Work out the finished part from the listing and answer in its coordinate system (mm). Face numbers are marked on the shaded views. A direction names the side the tool comes from. Round coordinates to 2 decimals unless told otherwise and drop trailing zeros. Order: outer loops, then holes, each group sorted by start corner. A loop starts at its lowest first (then second) coordinate and runs counter-clockwise, first axis right, second up. Notation, with made-up numbers: (-25, 62) -> (-5, 62) arc R6 ccw to (-5, 70) -> close; hole circle Ø9 at (66.5, 41.25). An arc over 180 degrees is marked (long way). Use one line per item in the form item = value.
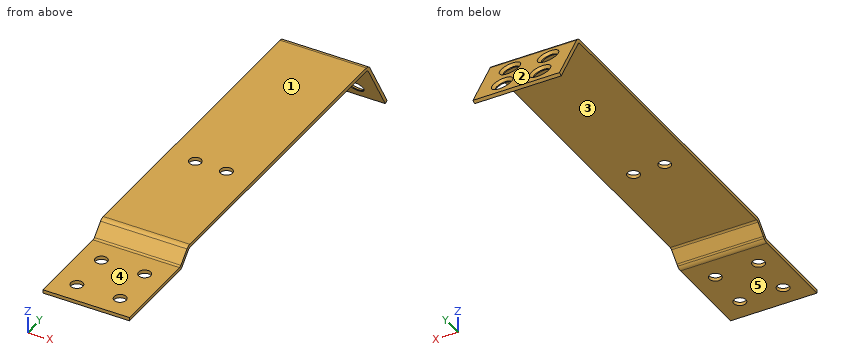
```python
from build123d import *

# Parameters (mm, degrees)
SKETCH_1_W                            = 50
SKETCH_1_H                            = 245
SM_BASE_FLANGE_1_DEPTH                = 2
SM_START                              = -25
SM_EDGE_FLANGE_1_DEPTH                = 50
SM_EDGE_FLANGE_1_2_DEPTH              = 50
OTHER_START                           = -25
OTHER_1_DEPTH                         = 50
OTHER_1_2_DEPTH                       = 50
HOLE_WIZARD_M61_D                     = 9
HOLE_WIZARD_M61_CSINK_D               = 12
HOLE_WIZARD_M61_CSINK_ANGLE           = 90
HOLE_WIZARD_M61_ON_FACE_2_D           = 9
HOLE_WIZARD_M61_ON_FACE_2_CSINK_D     = 12
HOLE_WIZARD_M61_ON_FACE_2_CSINK_ANGLE = 90
HOLE_WIZARD_M61_ON_FACE_3_D           = 9
HOLE_WIZARD_M61_ON_FACE_3_CSINK_D     = 12
HOLE_WIZARD_M61_ON_FACE_3_CSINK_ANGLE = 90
SKETCH_9_R                            = 3.5
CUT_EXTRUDE_1_DEPTH                   = 2
SKETCH_10_R                           = 3.5
CUT_EXTRUDE_2_DEPTH                   = 2


# Read off the part's stored shape, not the designer's step: Ребро-кромка1, Изгиб1
# Sheet-metal steps are written as plain solids
with BuildPart() as part:
    # Sketch 1 → Базовая кромка1 (new body)
    with BuildSketch(Plane.XY):
        with Locations((0, 122.5)):
            Rectangle(SKETCH_1_W, SKETCH_1_H)
    extrude(amount=SM_BASE_FLANGE_1_DEPTH)

    # Ребро-кромка1 outline → Ребро-кромка1 (cut)
    with BuildSketch(Plane.YZ.offset(SM_START)):
        with BuildLine():
            ThreePointArc((241.535898385, 2), (243.535898385, 1.464101615), (245, 0))
            Line((245, 0), (245, 2))
            Line((245, 2), (241.535898385, 2))
        make_face()
    extrude(amount=SM_EDGE_FLANGE_1_DEPTH, mode=Mode.SUBTRACT)

    # Sm Edge Flange 1 2 outline → Sm Edge Flange 1 2 (add)
    with BuildSketch(Plane.YZ.offset(SM_START)):
        with BuildLine():
            Line((262.422649731, -30.176914536), (245, 0))
            Line((245, 0), (241.535898385, 0))
            ThreePointArc((241.535898385, 0), (242.535898385, -0.267949192), (243.267949192, -1))
            Line((243.267949192, -1), (260.690598923, -31.176914536))
            Line((260.690598923, -31.176914536), (262.422649731, -30.176914536))
        make_face()
    extrude(amount=SM_EDGE_FLANGE_1_2_DEPTH)

    # Other 1 outline → Other 1 (cut)
    with BuildSketch(Plane.YZ.offset(OTHER_START)):
        with BuildLine():
            Line((241.535898385, 2), (54.65685425, 2))
            Line((54.65685425, 2), (53.82842715, 1.17157285))
            ThreePointArc((53.82842715, 1.17157285), (52.530733743, 0.304481837), (51, -3.6e-08))
            Line((51, -3.6e-08), (241.535898385, 0))
            ThreePointArc((241.535898385, 0), (242.535898385, -0.267949192), (243.267949192, -1))
            Line((243.267949192, -1), (260.690598923, -31.176914536))
            Line((260.690598923, -31.176914536), (262.422649731, -30.176914536))
            Line((262.422649731, -30.176914536), (245, 0))
            ThreePointArc((245, 0), (243.535898385, 1.464101615), (241.535898385, 2))
        make_face()
    extrude(amount=OTHER_1_DEPTH, mode=Mode.SUBTRACT)

    # Other 1 2 outline → Other 1 2 (add)
    with BuildSketch(Plane.YZ.offset(OTHER_START)):
        with BuildLine():
            Line((241.535898385, 10), (61.485281398, 10.000000033))
            ThreePointArc((61.485281398, 10.000000033), (59.954547643, 9.695518165), (58.656854226, 8.828427148))
            Line((58.656854226, 8.828427148), (52.414213588, 2.585786412))
            ThreePointArc((52.414213588, 2.585786412), (51.765366878, 2.152240902), (51, 1.999999964))
            Line((51, 1.999999964), (54.65685425, 2))
            Line((54.65685425, 2), (60.071067788, 7.414213586))
            ThreePointArc((60.071067788, 7.414213586), (60.719914496, 7.847759096), (61.485281374, 8.000000033))
            Line((61.485281374, 8.000000033), (241.535898385, 8))
            ThreePointArc((241.535898385, 8), (242.535898385, 7.732050808), (243.267949192, 7))
            Line((243.267949192, 7), (260.690598923, -23.176914536))
            Line((260.690598923, -23.176914536), (262.422649731, -22.176914536))
            Line((262.422649731, -22.176914536), (245, 8))
            ThreePointArc((245, 8), (243.535898385, 9.464101615), (241.535898385, 10))
        make_face()
    extrude(amount=OTHER_1_2_DEPTH)

    # Зенковка для винта с потайной головкой M61 (through all)
    with Locations(Plane(origin=(-11, 257.422649731, -13.516660498), x_dir=(0, -0.5, 0.866025403784), z_dir=(0, 0.866025403784, 0.5))):
        with Locations((0, 0)):
            CounterSinkHole(HOLE_WIZARD_M61_D / 2, HOLE_WIZARD_M61_CSINK_D / 2, counter_sink_angle=HOLE_WIZARD_M61_CSINK_ANGLE)

    # Зенковка для винта с потайной головкой M61 on face 2 (through all)
    with Locations(Plane(origin=(11, 257.422649731, -13.516660498), x_dir=(0, -0.500000174844, 0.866025302838), z_dir=(0, 0.866025302838, 0.500000174844))):
        with Locations((0, 0)):
            CounterSinkHole(HOLE_WIZARD_M61_ON_FACE_2_D / 2, HOLE_WIZARD_M61_ON_FACE_2_CSINK_D / 2, counter_sink_angle=HOLE_WIZARD_M61_ON_FACE_2_CSINK_ANGLE)

    # Зенковка для винта с потайной головкой M61 on face 3 (through all)
    with Locations(Plane(origin=(11, 249.422649731, 0.339745962), x_dir=(0, -0.500000174844, 0.866025302838), z_dir=(0, 0.866025302838, 0.500000174844))):
        with Locations((0, 0), (0, -22)):
            CounterSinkHole(HOLE_WIZARD_M61_ON_FACE_3_D / 2, HOLE_WIZARD_M61_ON_FACE_3_CSINK_D / 2, counter_sink_angle=HOLE_WIZARD_M61_ON_FACE_3_CSINK_ANGLE)

    # Эскиз9 → Вытянуть1 (cut)
    with BuildSketch(Plane.XY.offset(2)):
        with Locations((-12.5, 37.5)):
            Circle(SKETCH_9_R)
        with Locations((-12.5, 12.5)):
            Circle(SKETCH_9_R)
        with Locations((12.5, 12.5)):
            Circle(SKETCH_9_R)
        with Locations((12.5, 37.5)):
            Circle(SKETCH_9_R)
    extrude(amount=-CUT_EXTRUDE_1_DEPTH, mode=Mode.SUBTRACT)

    # Эскиз10 → Вытянуть2 (cut)
    with BuildSketch(Plane.XY.offset(10)):
        with Locations((-9, 127)):
            Circle(SKETCH_10_R)
        with Locations((9, 127)):
            Circle(SKETCH_10_R)
    extrude(amount=-CUT_EXTRUDE_2_DEPTH, mode=Mode.SUBTRACT)


solid = part.part
```
Item 1: Consider line 1 along X through (y, z) = (12, 1); line 2 along Y through (x, z) = (-12, 1); line 3 along Y through (x, z) = (12.5, 0.65). Determine where each line is inside the solid, lowest interval first.
Findings:
line_1 = -25 to -15.96, -9.04 to 9.04, 15.96 to 25
line_2 = 0 to 9.04, 15.96 to 34.04, 40.96 to 53.65
line_3 = 0 to 9, 16 to 34, 41 to 53.19
Item 2: The part is cut by section A-A, the plane y = 37.5. Give the vertices of the cut face in (x, z), and give its area (3 significant figures).
Findings:
outline = (-25, 0) -> (-16, 0) -> (-16, 2) -> (-25, 2) -> close; (-9, 0) -> (9, 0) -> (9, 2) -> (-9, 2) -> close; (16, 0) -> (25, 0) -> (25, 2) -> (16, 2) -> close
area = 72.0 mm^2
Item 3: Determine the mould class of the marked faces 1, 2 and 3 for opening direction Y: released by +Y, released by -Y, zero draft, split by the parting line, or undercut.
Findings:
face_1 = zero draft
face_2 = released by +Y
face_3 = undercut
Item 4: Flat-ended cylindrical pins translate along their axes: P1, Ø1.5, axis at x = 7, y = 34, coming from the -Z side; P2, Ø6.5, axis at x = 12.5, y = 12.5, coming from the +Z side; P3, Ø1.5, axis at x = -3, z = 4, coming from the -Y side; P4, Ø6, axis at x = 5, z = -14.5, coming from the -Y side. Find the tip coordinate at first contact, or state that the pin passes through.
Findings:
P1 = 0
P2 = through
P3 = 53.08
P4 = 253.95
Item 5: For the marked faces 4 and 5, determine the directions among +Z, -Z, +X, -X, +Y, -Y from which every point of the face is accessible in a straight line to the end or side of a thin tool.
Findings:
face_4 = +Z, +X, -X, -Y
face_5 = -Z, +X, -X, -Y
Item 6: The part is cut by section C-C, the plane y = 180.5. Give the vertices of the cut face in (x, z).
Findings:
outline = (-25, 8) -> (25, 8) -> (25, 10) -> (-25, 10) -> close
Item 7: The part is cut by section B-B, the plane x = 20. Give the vertices of the cut face in (y, z).
Findings:
outline = (0, 0) -> (51, 0) arc R4 ccw to (53.83, 1.17) -> (60.07, 7.41) arc R2 cw to (61.49, 8) -> (241.54, 8) arc R2 cw to (243.27, 7) -> (260.69, -23.18) -> (262.42, -22.18) -> (245, 8) arc R4 ccw to (241.54, 10) -> (61.49, 10) arc R4 ccw to (58.66, 8.83) -> (52.41, 2.59) arc R2 cw to (51, 2) -> (0, 2) -> close
